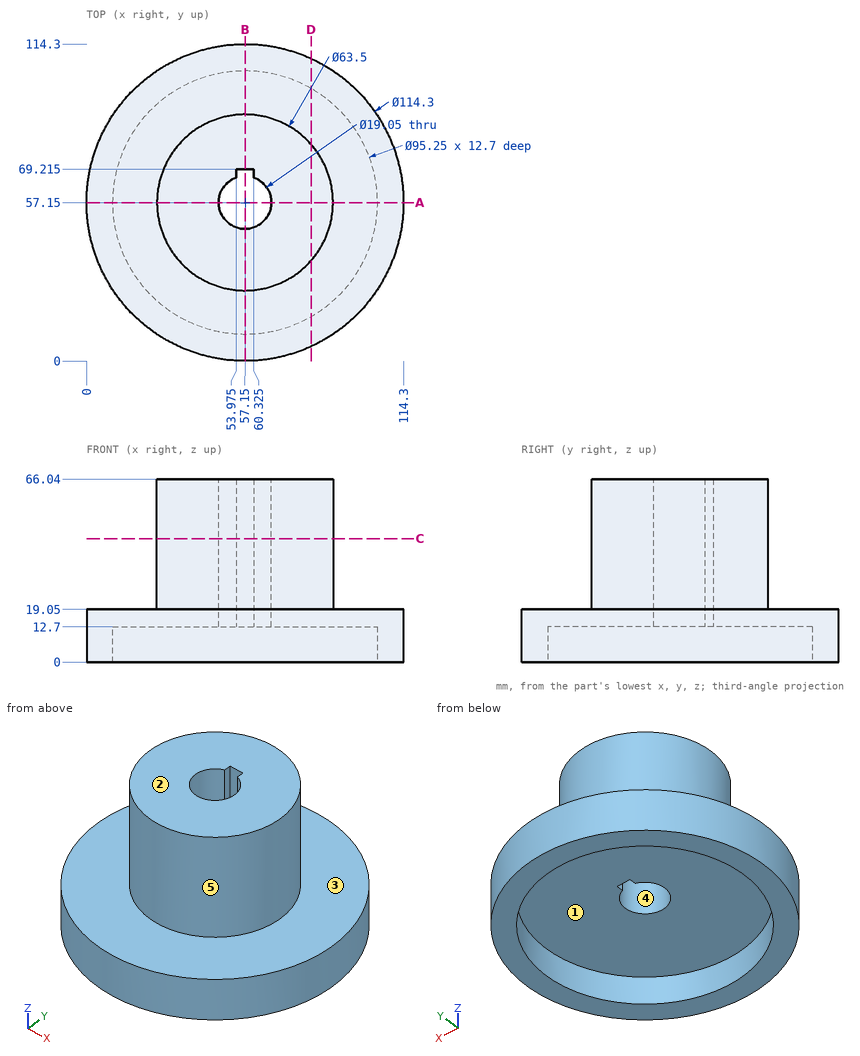
Job drawing, mm, ordinate dimensions from the low corner. One solid piece. A direction names the side the tool comes from. Give positions to 0.01 mm unless a question says otherwise; leave off trailing zeros. Order: outer loops, then holes, each group sorted by start corner. A loop starts at its lowest first (then second) coordinate and runs counter-clockwise, first axis right, second up. Notation, with made-up numbers: (78.5, -26.75) - (125.5, -26.75) arc R10 ccw to (125.5, -9.75) - close; hole circle Ø7 at (-40, 6.25). An arc over 180 degrees is marked (long way). Return JSON: item names as keys, results as strings.
1) Cut at C-C, the plane z = 44.5. Give the cut face in (x, y) (3 decimals), plus the area to 3 significant figures.
Geometry says:
{"outline": "circle Ø63.5 at (57.15, 57.15); hole (53.975, 66.13) arc R9.525 ccw (long way) to (60.325, 66.13) - (60.325, 69.215) - (53.975, 69.215) - close", "area": "2,860 mm²"}
2) 3-axis set-ups, long thin cutter, end or side, ignore diameter. For the marked faces 1 and 2: which of +Z, -Z, +X, -X, +Y, -Y reach the whole face in a straight line?
Geometry says:
{"face 1": "-Z", "face 2": "+Z, +X, -X, +Y, -Y"}
3) Pull direction Y, two halves, no side cores. Call the marked faces 3, 4 and 5: pulls with the +Y half, pulls with the -Y half, needs draft (parallel to the pull), parting line crosses it, or undercut.
Geometry says:
{"face 3": "needs draft", "face 4": "undercut", "face 5": "parting line crosses it"}
4) Cut at D-D, the plane x = 81. Give the cut face in (y, z).
Geometry says:
{"outline": "(5.21, 0) - (15.93, 0) - (15.93, 12.7) - (98.37, 12.7) - (98.37, 0) - (109.09, 0) - (109.09, 19.05) - (78.11, 19.05) - (78.11, 66.04) - (36.19, 66.04) - (36.19, 19.05) - (5.21, 19.05) - close"}
5) Flat gauge pins, fed straight in: P1, Ø2, axis at x = 58.5, y = 102, coming from the -Z side; P2, Ø6, axis at x = 28.5, z = 47.5, coming from the -Y side; P3, Ø2.5, axis at y = 68, z = 42, coming from the -X side; P4, Ø11.5, axis at x = 57.15, y = 57.15, coming from the +Z side. Where does each tip first touch, or does it go through?
Geometry says:
{"P1": "z = 12.7", "P2": "y = 38.44", "P3": "x = 26.89", "P4": "through"}
6) Cut at A-A, the plane y = 57.15. Give the cut face in (x, z) (3 decimals).
Geometry says:
{"outline": "(0, 0) - (9.525, 0) - (9.525, 12.7) - (47.625, 12.7) - (47.625, 66.04) - (25.4, 66.04) - (25.4, 19.05) - (0, 19.05) - close; (66.675, 12.7) - (104.775, 12.7) - (104.775, 0) - (114.3, 0) - (114.3, 19.05) - (88.9, 19.05) - (88.9, 66.04) - (66.675, 66.04) - close"}
7) Cut at B-B, the plane x = 57.15. Give the cut face in (y, z) (3 decimals).
Geometry says:
{"outline": "(0, 0) - (9.525, 0) - (9.525, 12.7) - (47.625, 12.7) - (47.625, 66.04) - (25.4, 66.04) - (25.4, 19.05) - (0, 19.05) - close; (69.215, 12.7) - (104.775, 12.7) - (104.775, 0) - (114.3, 0) - (114.3, 19.05) - (88.9, 19.05) - (88.9, 66.04) - (69.215, 66.04) - close"}
8) Probe line 1 (Y direction, x = 57, z = 6); line 2 (Y direction, x = 57.15, z = 27) (3 decimals); line 3 (X direction, y = 57, z = 44). List the from-to ranges inside material, lowest first. Write a range as from..to.
Geometry says:
{"line 1": "0..9.53, 104.77..114.3", "line 2": "25.4..47.625, 69.215..88.9", "line 3": "25.4..47.63, 66.67..88.9"}
